from build123d import *

# Parameters (mm, degrees)
F1_DEPTH  = 57.15
F3_DEPTH  = 7.9375
F5_DEPTH  = 7.9375
F6_R      = 9.92251
F7_DEPTH  = 88.901
F8_W      = 53.975
F8_H      = 44.45
F9_DEPTH  = 7.9375
F10_R     = 10.3251
F11_DEPTH = 7.9385
F12_R     = 4.7625
F13_R     = 12.7
F14_R     = 6.35


with BuildPart() as f1:
    # F0 (on Right) → F1 (new body)
    with BuildSketch(Plane.YZ):
        Polygon((0, 44.45), (0, 0), (88.9, 0), (88.9, 44.45), (80.9625, 44.45), (80.9625, 7.9375), (7.9375, 7.9375), (7.9375, 44.45), align=None)
    extrude(amount=F1_DEPTH)

    # F2 (on face) → F3 (join)
    with BuildSketch(Plane.XZ):
        with BuildLine():
            Line((0, 44.45), (57.15, 44.45))
            ThreePointArc((57.15, 44.45), (28.575, 73.025), (0, 44.45))
        make_face()
    extrude(amount=-F3_DEPTH)

    # F4 (on face) → F5 (join)
    with BuildSketch(Plane(origin=(0, 88.9, 0), x_dir=(-1, 0, 0), z_dir=(0, 1, 0))):
        with BuildLine():
            Line((-57.15, 44.45), (0, 44.45))
            ThreePointArc((0, 44.45), (-28.575, 73.025), (-57.15, 44.45))
        make_face()
    extrude(amount=-F5_DEPTH)

    # F6 (on face) → F7 (cut, through all)
    with BuildSketch(Plane.XZ):
        with Locations((28.575, 44.45)):
            Circle(F6_R)
    extrude(amount=-F7_DEPTH, mode=Mode.SUBTRACT)

    # F8 (on face) → F9 (join)
    with BuildSketch(Plane.XY.offset(7.9375)):
        with Locations((84.1375, 44.45)):
            Rectangle(F8_W, F8_H)
        with BuildLine():
            Line((111.125, 66.675), (111.125, 22.225))
            ThreePointArc((111.125, 22.225), (133.35, 44.45), (111.125, 66.675))
        make_face()
    extrude(amount=-F9_DEPTH)

    # F10 (on face) → F11 (cut, through all)
    with BuildSketch(Plane.XY.offset(7.9375)):
        with Locations((73.025, 44.45)):
            Circle(F10_R)
        with Locations((111.125, 44.45)):
            Circle(F10_R)
    extrude(amount=-F11_DEPTH, mode=Mode.SUBTRACT)

    # F12
    f12_edges = [f1.edges().sort_by_distance(p)[0] for p in [
        (28.575, 80.9625, 7.9375),
        (28.575, 7.9375, 7.9375),
    ]]
    fillet(f12_edges, radius=F12_R)

    # F13
    f13_edges = [f1.edges().sort_by_distance(p)[0] for p in [
        (28.575, 0, 0),
        (28.575, 88.9, 0),
    ]]
    fillet(f13_edges, radius=F13_R)

    # F14
    f14_edges = [f1.edges().sort_by_distance(p)[0] for p in [
        (57.15, 66.675, 3.96875),
        (57.15, 22.225, 3.96875),
    ]]
    fillet(f14_edges, radius=F14_R)


solid = f1.part
The model under review builds one solid part; all positions refer to its coordinate system, in mm. A direction names the side the tool comes from. Round coordinates to 2 decimals unless told otherwise and drop trailing zeros. Write each loop counter-clockwise with the first axis right and the second up, starting at its lowest first coordinate (ties: lowest second). Pieces come first, ordered by that corner, then holes. Notation, with made-up numbers: M -36,85.25 L 0,85.25 A18 ccw 0,115.25 Z; hole C 89,44 d7. An arc over 180 degrees is marked long. Use a Markdown table: item, result. Add a question column.
Q1. Insertion check: pin 1 (6.5 mm diameter, centred on x = 85, z = 2.5, fed in from -Y) (3 decimals); pin 2 (5 mm diameter, centred on y = 4, z = 27.5, fed in from +X); pin 3 (12.5 mm diameter, centred on x = 111.125, y = 44.45, fed in from -Z); pin 4 (10 mm diameter, centred on x = 104, y = 58, fed in from +Z). Each pin has a flat end and moves straight along its axis. Give the tip position at first contact, or say it passes through.
Q2. The part is to be moulded in two halves that separate along X. For faces 4 (the face through (26.424, 84.876, 34.763)), 5 (the face through (26.424, 3.913, 34.763)), 6 (the face through (28.98, 3.82, 3.62)), 7 (the face through (58.961, 20.315, 3.913)), say which applies: pulls with the +X half, pulls with the -X half, needs draft (parallel to the pull), parting line crosses it, or undercut.
Q3. We need section A-A, the plane z = 29. State the section outline as (x, y) points, plus the area to 3 significant figures.
Q4. Machinability: for faces 1 (the face through (28.975, 79.604, 9.37)), 2 (the face through (87, 22.225, 4)), 3 (the face through (87, 66.675, 4)), which of the approach directions +Z, -Z, +X, -X, +Y, -Y give a long, thin tool a straight path to every point of the face, cutting with its end or side? Answer none if there is none.
Q5. We need section C-C, the plane x = 31.5. State the section outline as (y, z) points (1 decimal), plus the area to 3 significant figures.
Q6. To check wall thickness, follow line 1 (X direction, y = 44, z = 3); line 2 (Y direction, x = 42, z = 64); line 3 (X direction, y = 3, z = 44). State the ranges of each line that lie inside material, in increasing order.
Q7. We need section D-D, the plane z = 49.5. State the section outline as (x, y) points.
Q8. We need section B-B, the plane y = 44.45. State the section outline as (x, z) points.
Findings below:
| question | item | result |
|---|---|---|
| 1 | pin 1 | stops at y = 22.225 |
| 1 | pin 2 | stops at x = 57.15 |
| 1 | pin 3 | passes through |
| 1 | pin 4 | stops at z = 7.94 |
| 2 | face 4 | undercut |
| 2 | face 5 | undercut |
| 2 | face 6 | needs draft |
| 2 | face 7 | pulls with the +X half |
| 3 | outline | M 0,0 L 57.15,0 L 57.15,7.94 L 0,7.94 Z; M 0,80.96 L 57.15,80.96 L 57.15,88.9 L 0,88.9 Z |
| 3 | area | 907 mm² |
| 4 | face 1 | +Z, +X, -X |
| 4 | face 2 | +Z, -Z, +X, -Y |
| 4 | face 3 | +Z, -Z, +X, +Y |
| 5 | outline | M 0,12.7 A12.7 ccw 12.7,0 L 76.2,0 A12.7 ccw 88.9,12.7 L 88.9,35 L 81,35 L 81,12.7 A4.8 cw 76.2,7.9 L 12.7,7.9 A4.8 cw 7.9,12.7 L 7.9,35 L 0,35 Z; M 0,53.9 L 7.9,53.9 L 7.9,72.9 L 0,72.9 Z; M 81,53.9 L 88.9,53.9 L 88.9,72.9 L 81,72.9 Z |
| 5 | area | 1,380 mm² |
| 6 | line 1 | x = 0 to 62.71, 83.34 to 100.81, 121.44 to 133.35 |
| 6 | line 2 | y = 0 to 7.94, 80.96 to 88.9 |
| 6 | line 3 | x = 0 to 18.66, 38.49 to 57.15 |
| 7 | outline | M 0.45,0 L 20.03,0 L 20.03,7.94 L 0.45,7.94 Z; M 0.45,80.96 L 20.03,80.96 L 20.03,88.9 L 0.45,88.9 Z; M 37.12,0 L 56.7,0 L 56.7,7.94 L 37.12,7.94 Z; M 37.12,80.96 L 56.7,80.96 L 56.7,88.9 L 37.12,88.9 Z |
| 8 | outline | M 0,0 L 62.7,0 L 62.7,7.94 L 0,7.94 Z; M 83.35,0 L 100.8,0 L 100.8,7.94 L 83.35,7.94 Z; M 121.45,0 L 133.35,0 L 133.35,7.94 L 121.45,7.94 Z |
